Drawing for the job (mm, zero at the part's lowest x, y, z). Round coordinates to 2 decimals unless told otherwise and drop trailing zeros. Order: outer loops, then holes, each group sorted by start corner. A loop starts at its lowest first (then second) coordinate and runs counter-clockwise, first axis right, second up. Notation, with made-up numbers: M 72,68 L 119,68 A26 cw 119,88 Z; hole C -23,25 d5. An arc over 180 degrees is marked long. Answer as CSV lines item,"result". Start each with the question number.
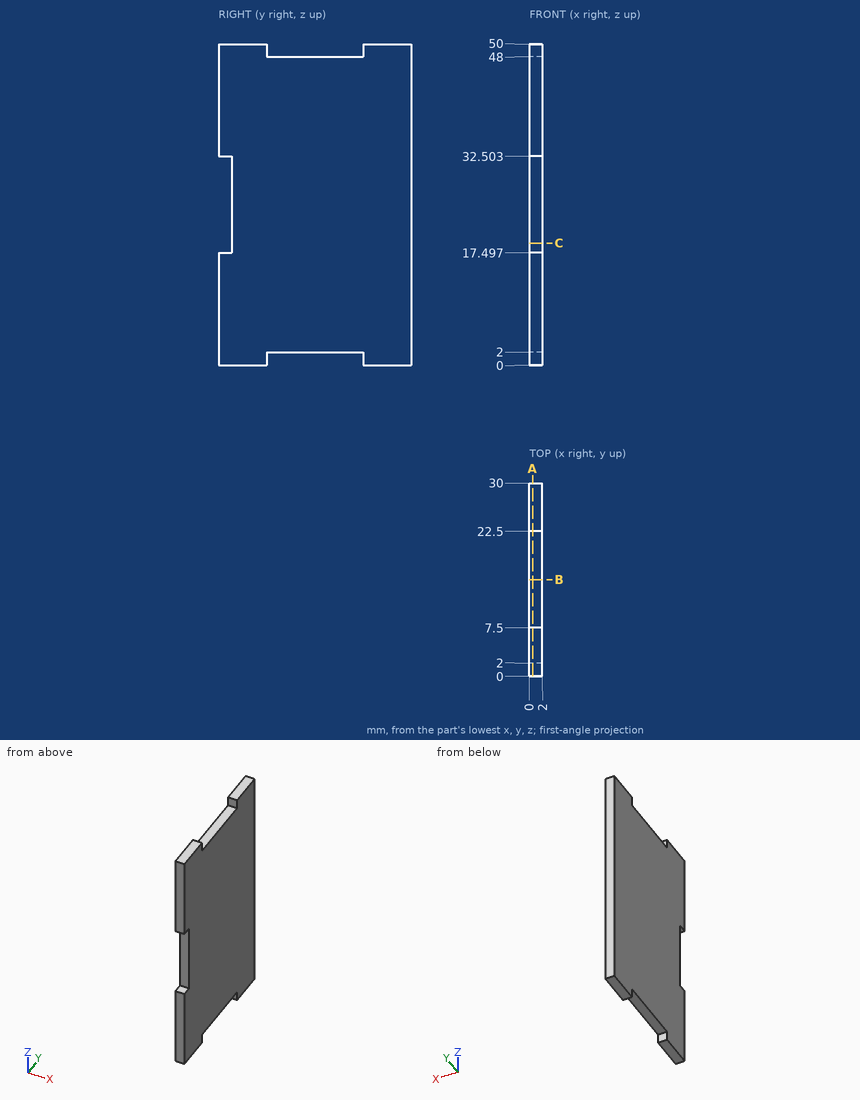
Q1. Band-saw the part on C-C, the plane z = 19. Write the cut outline in (x, y).
Q2. Band-saw the part on B-B, the plane y = 15. Write the cut outline in (x, z).
Q3. Probe line 1 along Z through (x, y) = (1.2, 1.5); line 2 along Y through (x, z) = (0.25, 26.5); line 3 along Z through (x, y) = (0.95, 13). List the from-to ranges inside material, lowest first. Write a range as from..to.
Q4. Drop flat-ended pins along their axis: P1, Ø0.6, axis at x = 1.5, y = 15.5, coming from the +Z side; P2, Ø1, axis at x = 1.5, z = 28, coming from the -Y side; P3, Ø1, axis at x = 1, y = 16, coming from the -Z side. Give the stop position or say it passes through.
Q5. Band-saw the part on A-A, the plane x = 0.5. Write the cut outline in (y, z), then the cut area to 3 significant figures.
Answer:
1,outline,"M 0,2 L 2,2 L 2,30 L 0,30 Z"
2,outline,"M 0,2 L 2,2 L 2,48 L 0,48 Z"
3,line 1,"z = 0..17.5, 32.5..50"
3,line 2,"y = 2..30"
3,line 3,"z = 2..48"
4,P1,"stops at z = 48"
4,P2,"stops at y = 2"
4,P3,"stops at z = 2"
5,outline,"M 0,0 L 7.5,0 L 7.5,2 L 22.5,2 L 22.5,0 L 30,0 L 30,50 L 22.5,50 L 22.5,48 L 7.5,48 L 7.5,50 L 0,50 L 0,32.5 L 2,32.5 L 2,17.5 L 0,17.5 Z"
5,area,"1,410 mm^2"
